Model file for the job. Use its own axes, mm. Face numbers are marked on the shaded views. A direction names the side the tool comes from. Round coordinates to 2 decimals unless told otherwise and drop trailing zeros. Order: outer loops, then holes, each group sorted by start corner. A loop starts at its lowest first (then second) coordinate and runs counter-clockwise, first axis right, second up. Notation, with made-up numbers: (38, -4.5) -> (53, -4.5) arc R27 ccw to (53, 16.5) -> close; hole circle Ø3 at (76, -11.5). An arc over 180 degrees is marked (long way). Answer as CSV lines item,"result".
```python
from build123d import *

# Parameters (mm, degrees)
F0_W        = 25.4
F0_H        = 76.2
F0_R        = 3.175
F1_DEPTH    = 25.4
F2_W        = 25.4
F2_H        = 25.4
F3_DEPTH    = 25.4
F4_W        = 17.78
F4_H        = 17.78
F5_DEPTH    = 63.5
F6_T1_DEPTH = 88.9
F6_T3_DEPTH = 88.9


# Not quite as in the source:
# - a fillet or chamfer that OpenCascade refuses, or shapes differently, is made with other operations: its cross-section is extruded or revolved along the edge and cut away or added


with BuildPart() as f1:
    # F0 (on Front) → F1 (new body)
    with BuildSketch(Plane.XZ):
        with Locations((1.0031497249, 16.5614479933)):
            Rectangle(F0_W, F0_H)
        with Locations((0, 29.2614479933)):
            Circle(F0_R, mode=Mode.SUBTRACT)
        with Locations((0, 41.9614479933)):
            Circle(F0_R, mode=Mode.SUBTRACT)
    extrude(amount=F1_DEPTH)

    # F2 (on face) → F3 (join)
    with BuildSketch(Plane.XZ.offset(25.4)):
        with Locations((1.0031497249, -8.8385520067)):
            Rectangle(F2_W, F2_H)
    extrude(amount=F3_DEPTH)

    # F4 (on face) → F5 (cut, symmetric)
    with BuildSketch(Plane(origin=(-11.6968502751, 0, 0), x_dir=(0, -1, 0), z_dir=(-1, 0, 0))):
        with Locations((38.1, -8.8385520067)):
            Rectangle(F4_W, F4_H)
    extrude(amount=F5_DEPTH, both=True, mode=Mode.SUBTRACT)

    # F6: fillet of radius 12.7 on 4 edges, made by hand

    # F6_s2 → F6_t1 (cut)
    with BuildSketch(Plane.YZ.offset(-43.4468502751)):
        with BuildLine():
            ThreePointArc((-50.8, -8.8385520067), (-47.0802561211, 0.1417041144), (-38.1, 3.8614479933))
            Line((-38.1, 3.8614479933), (-50.8, 3.8614479933))
            Line((-50.8, 3.8614479933), (-50.8, -8.8385520067))
        make_face()
        with BuildLine():
            ThreePointArc((-38.1, -21.5385520067), (-47.0802561211, -17.8188081278), (-50.8, -8.8385520067))
            Line((-50.8, -8.8385520067), (-50.8, -21.5385520067))
            Line((-50.8, -21.5385520067), (-38.1, -21.5385520067))
        make_face()
    extrude(amount=F6_T1_DEPTH, mode=Mode.SUBTRACT)

    # F6_s4 → F6_t3 (cut)
    with BuildSketch(Plane.XY.offset(-53.2885520067)):
        with BuildLine():
            ThreePointArc((1.0031497249, -50.8), (-7.9771063962, -47.0802561211), (-11.6968502751, -38.1))
            Line((-11.6968502751, -38.1), (-11.6968502751, -50.8))
            Line((-11.6968502751, -50.8), (1.0031497249, -50.8))
        make_face()
        with BuildLine():
            ThreePointArc((13.7031497249, -38.1), (9.983405846, -47.0802561211), (1.0031497249, -50.8))
            Line((1.0031497249, -50.8), (13.7031497249, -50.8))
            Line((13.7031497249, -50.8), (13.7031497249, -38.1))
        make_face()
    extrude(amount=F6_T3_DEPTH, mode=Mode.SUBTRACT)


solid = f1.part
```
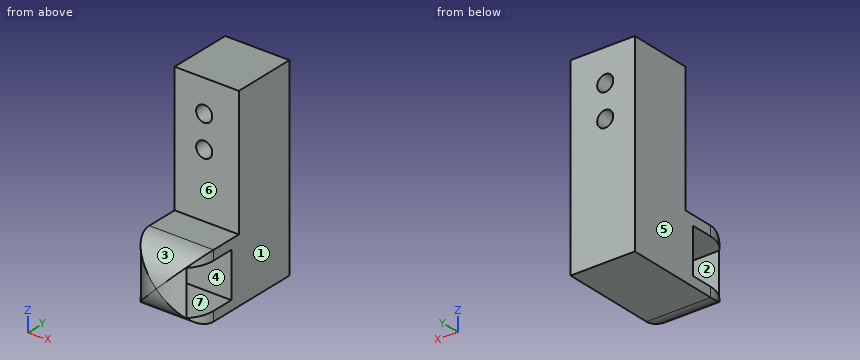
Q1. Tool access for the marked faces 5, 6 and 7: list every direction of +Z, -Z, +X, -X, +Y, -Y with a clear straight run to the whole face (end or side of a thin tool).
Checks:
face 5,"+Z, -Z, -X, +Y, -Y"
face 6,"+Z, +X, -X, -Y"
face 7,"+X, -X"
Q2. Wall check: L1, parallel to Z at x = 0, y = -6.5; L2, parallel to Y at x = 6.25, z = 34.5; L3, parallel to Y at x = 10.25, z = -12. Give the ranges that are in metal, low to high. Write a range as [from, to].
Checks:
L1,"[-21.54, 26.09], [32.44, 38.79], [45.14, 54.66]"
L2,"[-25.4, 0]"
L3,"[-29.21, 0]"
Q3. Saw through at A-A (x = 0). Write the cut outline in (y, z).
Checks:
outline,"(-50.76, -9.84) arc R12.7 ccw to (-38.1, -21.54) -> (0, -21.54) -> (0, 26.09) -> (-25.4, 26.09) -> (-25.4, 3.86) -> (-38.1, 3.86) arc R12.7 ccw to (-50.76, -7.84) -> close; (-25.4, 32.44) -> (0, 32.44) -> (0, 38.79) -> (-25.4, 38.79) -> close; (-25.4, 45.14) -> (0, 45.14) -> (0, 54.66) -> (-25.4, 54.66) -> close; hole (-46.99, -17.73) -> (-29.21, -17.73) -> (-29.21, 0.05) -> (-46.99, 0.05) -> close"
Q4. Saw through at D-D (y = -22.5). Write the cut outline in (x, z) (3 decimals), plus the area to 3 significant figures.
Checks:
outline,"(-11.697, -21.539) -> (13.703, -21.539) -> (13.703, 54.661) -> (-11.697, 54.661) -> close; hole circle Ø6.35 at (0, 29.261); hole circle Ø6.35 at (0, 41.961)"
area,"1,870 mm²"
Q5. Saw through at C-C (x = 7.75). Write the cut outline in (y, z).
Checks:
outline,"(-48.86, -15.59) arc R12.7 ccw to (-38.1, -21.54) -> (0, -21.54) -> (0, 54.66) -> (-25.4, 54.66) -> (-25.4, 3.86) -> (-38.1, 3.86) arc R12.7 ccw to (-48.86, -2.09) -> close; hole (-46.99, -17.73) -> (-29.21, -17.73) -> (-29.21, 0.05) -> (-46.99, 0.05) -> close"
Q6. Flat gauge pins, fed straight in: pin 1 (5 mm diameter, centred on x = -4, z = 31, fed in from +Y); pin 2 (14 mm diameter, centred on x = 6, y = -37.5, fed in from +Z); pin 3 (12 mm diameter, centred on y = -37, z = -9, fed in from +X). Where does each tip first touch, or does it go through?
Checks:
pin 1,"y = 0"
pin 2,"z = 3.86"
pin 3,"through"
Q7. Saw through at B-B (z = -7.5). Write the cut outline in (x, y).
Checks:
outline,"(-11.7, -29.21) -> (13.7, -29.21) -> (13.7, 0) -> (-11.7, 0) -> close; (-8.07, -46.99) arc R12.7 ccw to (-0.34, -50.73) -> (2.34, -50.73) arc R12.7 ccw to (10.07, -46.99) -> close"
Q8. Mould opens along Z. For the marked faces 1, 2, 3 and 4 say: +Z half, -Z half, draft (parallel to the pull), parting line (faces both ways), or undercut.
Checks:
face 1,"draft"
face 2,"undercut"
face 3,"+Z half"
face 4,"undercut"
